Model file for the job. Use its own axes, mm. A direction names the side the tool comes from. Give positions to 0.01 mm unless a question says otherwise; leave off trailing zeros. Loops run counter-clockwise (first coordinate to the right, second up) from the corner with the lowest first, then second, coordinate; pieces in that order, holes last. Notation, with made-up numbers: M 19.5,-29 L 56.5,-29 A7 ccw 56.5,-21 Z; hole C -5,-24 d2. An arc over 180 degrees is marked long. Answer in a Markdown table with one row per item.
```python
from build123d import *

# Parameters (mm, degrees)
F0_W     = 200
F0_H     = 250
F1_DEPTH = 200
F2_W     = 180
F2_H     = 230
F3_DEPTH = 190
F4_DEPTH = 180
F0_H_2   = 100
F5_DEPTH = 10


with BuildPart() as f1:
    # F0 (on Top) → F1 (new body)
    with BuildSketch(Plane.XY):
        with Locations((40.9984113305, 1.9545629621)):
            Rectangle(F0_W, F0_H)
    extrude(amount=F1_DEPTH)

    # F2 (on face) → F3 (cut)
    with BuildSketch(Plane.XY.offset(200)):
        with Locations((40.9984113305, 1.9545629621)):
            Rectangle(F2_W, F2_H)
    extrude(amount=-F3_DEPTH, mode=Mode.SUBTRACT)

    # F4 (cut): a face of the model
    f4_faces = [f1.faces().sort_by_distance(p)[0] for p in [
        (-55.8000265508, 1.9545629621, 200),
    ]]
    extrude(f4_faces, amount=-F4_DEPTH, mode=Mode.SUBTRACT)

    # F0 (on Top) → F5 (join)
    with BuildSketch(Plane.XY):
        with Locations((40.9984113305, -173.0454370379)):
            Rectangle(F0_W, F0_H_2)
    extrude(amount=F5_DEPTH)


solid = f1.part
```
(1) Saw through at D-D, the plane y = -202. Give the cut face in (x, z).
Established:
| item | result |
|---|---|
| outline | M -59,0 L 141,0 L 141,10 L -59,10 Z |
(2) Which spindle directions (+Z, -Z, +X, -X, +Y, -Y) get a long thin tool onto all of the face, cutting with end or side? Do faces 4 (the flat face through (40, -123.045, 15)), 5 (the flat face through (130.998, 0, 15)), 6 (the flat face through (40, -46, 0)). Say none if no direction does.
Established:
| item | result |
|---|---|
| face 4 | +Z, +X, -X, -Y |
| face 5 | +Z |
| face 6 | -Z, +X, -X, +Y, -Y |
(3) Mould opens along Y. For faces 1 (the flat face through (40, -223.045, 5)), 2 (the flat face through (40, -172, 10)), 3 (the flat face through (-49.002, 0, 15)) say: pulls with the +Y half, pulls with the -Y half, needs draft (parallel to the pull), parting line crosses it, or undercut.
Established:
| item | result |
|---|---|
| face 1 | pulls with the -Y half |
| face 2 | needs draft |
| face 3 | undercut |
(4) Saw through at B-B, the plane y = 79. Give the cut face in (x, z), and give its area (3 significant figures).
Established:
| item | result |
|---|---|
| outline | M -59,0 L 141,0 L 141,20 L 131,20 L 131,10 L -49,10 L -49,20 L -59,20 Z |
| area | 2,200 mm2 |
(5) Saw through at A-A, the plane z = 14.75. Give the cut face in (x, y), and give its area (3 significant figures).
Established:
| item | result |
|---|---|
| outline | M -59,-123.05 L 141,-123.05 L 141,126.95 L -59,126.95 Z; hole M -49,-113.05 L 131,-113.05 L 131,116.95 L -49,116.95 Z |
| area | 8,600 mm2 |
(6) Flat gauge pins, fed straight in: P1, Ø11, axis at x = 77.5, z = 16.5, coming from the -Y side; P2, Ø5, axis at x = 34, y = 82.5, coming from the +Z side. Where does each tip first touch, or does it go through?
Established:
| item | result |
|---|---|
| P1 | stops at y = -123.05 |
| P2 | stops at z = 10 |
(7) Wall check: L1, parallel to Y at x = -35.5, z = 10.5; L2, parallel to Z at x = 9.5, y = -50.5; L3, parallel to X at y = 77, z = 18.5. Give the ranges that are in metal, low to high.
Established:
| item | result |
|---|---|
| L1 | y = -123.05 to -113.05, 116.95 to 126.95 |
| L2 | z = 0 to 10 |
| L3 | x = -59 to -49, 131 to 141 |
(8) Saw through at C-C, the plane x = 107.5. Give the cut face in (y, z), and give its area (3 significant figures).
Established:
| item | result |
|---|---|
| outline | M -223.05,0 L 126.95,0 L 126.95,20 L 116.95,20 L 116.95,10 L -113.05,10 L -113.05,20 L -123.05,20 L -123.05,10 L -223.05,10 Z |
| area | 3,700 mm2 |
